Autodesk Inventor part; units mm, degrees
ref_plane "YZ Plane" through (0, 0, 0) normal (1, 0, 0) x (0, 1, 0)
ref_plane "XZ Plane" through (0, 0, 0) normal (0, 1, 0) x (-1, 0, 0)
ref_plane "XY Plane" through (0, 0, 0) normal (0, 0, 1) x (1, 0, 0)
sketch "Sketch1" plane through (0, 0, 0) normal (0, 0, 1) x (1, 0, 0)
  line L0 (0, 0) -> (175, 0)
  line L1 (175, 0) -> (175, 175)
  line L2 (175, 175) -> (0, 175)
  line L3 (0, 175) -> (0, 0)
  dimension "d0" = 175
  dimension "d1" = 175
extrude "Extrusion1" add sketch "Sketch1" along normal blind 100
sketch "Sketch2" plane through (0, 175, 0) normal (0, 1, 0) x (1, 0, 0)
  line L0 (0, 0) -> (175, 0)
  line L1 (0, -100) -> (175, -100)
  line L2 (0, 0) -> (175, 0)
  line L3 (175, 0) -> (175, -100)
  line L4 (175, -100) -> (0, -100)
  line L5 (0, -100) -> (0, 0)
  line L6 (10, -10) -> (165, -10)
  line L7 (165, -10) -> (165, -90)
  line L8 (165, -90) -> (10, -90)
  line L9 (10, -90) -> (10, -10)
  dimension "d4" = 10
  dimension "d5" = 10
  dimension "d6" = 10
  dimension "d7" = 10
extrude "Extrusion2" add sketch "Sketch2" along normal blind 10
sketch "Sketch3" plane through (10, 175, 10) normal (0, 1, 0) x (1, 0, 0)
  line L0 (0, -80) -> (0, 0)
  line L1 (0, -80) -> (155, -80)
  line L2 (0, 0) -> (155, 0)
  line L3 (155, 0) -> (155, -80)
  line L4 (155, -80) -> (0, -80)
  line L5 (0, -80) -> (0, 0)
  point P0 (-10, 10)
extrude "Extrusion3" cut sketch "Sketch3" against normal blind 9000
sketch "Sketch4" plane through (0, 0, 100) normal (0, 0, 1) x (1, 0, 0)
  line L0 (175, 0) -> (175, 185)
  line L1 (175, 185) -> (195, 185)
  line L2 (195, 185) -> (195, 0)
  line L3 (195, 0) -> (175, 0)
  line L4 (175, 0) -> (175, 185)
  point P0 (0, 0)
  dimension "d12" = 20
extrude "Extrusion4" add sketch "Sketch4" against normal blind 100
sketch "Sketch5" plane through (0, 0, 100) normal (0, 0, 1) x (1, 0, 0)
  line L0 (10, 175) -> (185, 175)
  line L1 (185, 175) -> (185, 10)
  line L2 (185, 10) -> (10, 10)
  line L3 (10, 10) -> (10, 175)
  line L4 (0, 185) -> (195, 185)
  line L5 (0, 0) -> (0, 185)
  line L6 (0, 0) -> (195, 0)
  line L7 (195, 0) -> (195, 185)
  dimension "d15" = 10
  dimension "d16" = 10
  dimension "d17" = 10
  dimension "d18" = 10
extrude "Extrusion5" cut sketch "Sketch5" against normal blind 100 contours L0 L1 L2 L3
sketch "Sketch6" plane through (195, 0, 100) normal (1, 0, 0) x (0, 0, -1)
  point P0 (100, 0)
sketch "Sketch7" plane through (0, 185, 0) normal (0, 1, 0) x (1, 0, 0)
  line L0 (0, -100) -> (195, -100)
  line L1 (0, 0) -> (195, 0)
  line L2 (195, 0) -> (195, -100)
  line L3 (195, -100) -> (0, -100)
  line L4 (0, -100) -> (0, 0)
extrude "Extrusion6" add sketch "Sketch7" along normal blind 10
sketch "Sketch8" plane through (0, 195, 0) normal (0, 1, 0) x (1, 0, 0)
  line L0 (10, -10) -> (10, 0)
  line L1 (10, -10) -> (185, -10)
  line L2 (185, -10) -> (185, -90)
  line L3 (185, -90) -> (10, -90)
  line L4 (10, -90) -> (10, -10)
  line L5 (0, -100) -> (195, -100)
  line L6 (195, -100) -> (195, 0)
  point P0 (0, 0)
  dimension "d23" = 10
  dimension "d24" = 10
extrude "Extrusion7" cut sketch "Sketch8" against normal blind 900
sketch "Sketch9" plane through (195, 0, 100) normal (1, 0, 0) x (0, 0, -1)
  line L0 (10, 185) -> (90, 185)
  line L1 (90, 185) -> (90, 10)
  line L2 (90, 10) -> (10, 10)
  line L3 (10, 10) -> (10, 185)
  line L4 (0, 195) -> (100, 195)
  line L5 (0, 0) -> (0, 195)
  line L6 (0, 0) -> (100, 0)
  line L7 (100, 0) -> (100, 195)
  dimension "d27" = 10
  dimension "d28" = 10
  dimension "d29" = 10
  dimension "d30" = 10
extrude "Extrusion8" cut sketch "Sketch9" against normal blind 900 contours L0 L1 L2 L3
sketch "Sketch10" plane through (0, 0, 100) normal (0, 0, 1) x (1, 0, 0)
  line L0 (185, 175) -> (10, 175)
  line L1 (185, 195) -> (185, 185)
  line L2 (10, 175) -> (185, 175)
  line L3 (185, 175) -> (185, 185)
  line L4 (185, 185) -> (10, 185)
  line L5 (10, 185) -> (10, 175)
  point P0 (0, 0)
extrude "Extrusion9" cut sketch "Sketch10" against normal blind 900
sketch "Sketch11" plane through (0, 0, 100) normal (0, 0, 1) x (1, 0, 0)
  line L0 (0, 0) -> (0, 195)
  line L1 (0, 0) -> (195, 0)
  line L2 (0, 195) -> (195, 195)
  line L3 (195, 195) -> (195, 0)
  line L4 (195, 0) -> (0, 0)
  line L5 (0, 0) -> (0, 195)
  line L6 (10, 185) -> (10, 10)
  line L7 (185, 10) -> (10, 10)
  line L8 (10, 185) -> (185, 185)
  line L9 (185, 185) -> (185, 10)
  line L10 (185, 10) -> (10, 10)
  line L11 (10, 10) -> (10, 185)
extrude "Extrusion10" add sketch "Sketch11" along normal blind 20
sketch "Sketch12" plane through (0, 195, 0) normal (0, 1, 0) x (1, 0, 0)
  line L0 (10, -90) -> (0, -90)
  line L1 (185, -120) -> (185, -90)
  line L2 (10, -90) -> (185, -90)
  line L3 (185, -90) -> (185, -110)
  line L4 (185, -110) -> (10, -110)
  line L5 (10, -110) -> (10, -90)
  line L6 (195, -120) -> (0, -120)
  point P0 (0, 0)
  dimension "d37" = 10
extrude "Extrusion11" cut sketch "Sketch12" against normal blind 900
sketch "Sketch13" plane through (195, 0, 0) normal (1, 0, 0) x (0, 0, -1)
  line L0 (-90, 185) -> (-10, 185)
  line L1 (-120, 10) -> (-110, 10)
  line L2 (-90, 185) -> (-110, 185)
  line L3 (-110, 185) -> (-110, 10)
  line L4 (-110, 10) -> (-90, 10)
  line L5 (-90, 10) -> (-90, 185)
  point P0 (0, 0)
extrude "Extrusion12" cut sketch "Sketch13" against normal blind 900
sketch "Sketch15" plane through (0, 10, 10) normal (0, 0, 1) x (1, 0, 0)
  line L0 (10, 175) -> (10, 0)
  line L1 (0, 115) -> (10, 115)
  line L2 (10, 115) -> (10, 105)
  line L3 (10, 105) -> (0, 105)
  line L4 (0, 105) -> (0, 115)
  point P0 (10, 115)
  point P1 (10, 115)
  dimension "d45" = 10
sketch "Sketch16" plane through (185, 10, 10) normal (0, 0, 1) x (1, 0, 0)
  line L0 (0, 115) -> (10, 115)
  line L1 (0, 115) -> (10, 115)
  line L2 (10, 115) -> (10, 105)
  line L3 (10, 105) -> (0, 105)
  line L4 (0, 105) -> (0, 115)
  point P0 (-185, -10)
  point P1 (10, 115)
  dimension "d46" = 10
properties part number "Battery housing"
The listing builds one solid part. Answer for the finished solid, in the listing's coordinates (mm). A direction names the side the tool comes from. Coordinates: 2 decimals unless noted, no trailing zeros. Write each loop counter-clockwise with the first axis right and the second up, starting at its lowest first coordinate (ties: lowest second). Pieces come first, ordered by that corner, then holes. Notation, with made-up numbers: (14, -34.75) - (54, -34.75) arc R8 cw to (54, -27.75) - close; hole circle Ø3 at (37, 7.25). An arc over 180 degrees is marked (long way). Return JSON: item names as keys, results as strings. Group by question number.
Q1. The part is cut by section A-A on x = 96.5. Write down the section's boundary in (y, z), and give its area (3 significant figures).
Q2. For a pull along Z with two mould halves and no side action, classify faces 1 (the flat face through (90, 191, 0)), 2 (the flat face through (185, 5, 59)), 3 (the flat face through (0, 90, 113)) as +Z half, -Z half, draft (parallel to the pull), parting line (faces both ways), or undercut.
Q3. The part is cut by section C-C on z = 112.5. Write down the section's boundary in (x, y), and give its area (3 significant figures).
Q4. Find the intervals of material crossed by line 1 along X through (y, z) = (25.5, 111.5); line 2 along Z through (x, y) = (9.5, 126.5), in increasing order. Write a range as [from, to].
Q5. Which of the six approach directions +Z, -Z, +X, -X, +Y, -Y give full straight-line access (tool end or side, diameter ignored) to faces 4 (the flat face through (185, 190, 59)), 5 (the flat face through (5, 99, 110)), 6 (the flat face through (10, 99, 115)), 7 (the flat face through (90, 4, 120))?
Evaluation:
{
 "1": {"outline": "(0, 0) - (10, 0) - (10, 10) - (0, 10) - close; (0, 110) - (10, 110) - (10, 120) - (0, 120) - close; (185, 0) - (195, 0) - (195, 10) - (185, 10) - close; (185, 110) - (195, 110) - (195, 120) - (185, 120) - close", "area": "400 mm2"},
 "2": {"face 1": "-Z half", "face 2": "undercut", "face 3": "draft"},
 "3": {"outline": "(0, 0) - (195, 0) - (195, 195) - (0, 195) - close; hole (10, 10) - (185, 10) - (185, 185) - (10, 185) - close", "area": "7,400 mm2"},
 "4": {"line 1": "x = [0, 10], [185, 195]", "line 2": "z = [0, 10], [110, 120]"},
 "5": {"face 4": "+Y, -Y", "face 5": "+X, -X", "face 6": "+Z, -Z", "face 7": "+Z, +X, -X, +Y, -Y"}
}
